```python
from build123d import *

# Parameters (mm, degrees)
SKETCH_1_R          = 10
EXTRUDE_1_DEPTH     = 5.5
SKETCH_2_R          = 6
EXTRUDE_2_DEPTH     = 5
SKETCH_3_R          = 3
EXTRUDE_3_DEPTH     = 1.5
SKETCH_4_R          = 4
EXTRUDE_4_DEPTH     = 10
CHAMFER_1_SIZE      = 1
SKETCH_5_W          = 2
SKETCH_5_H          = 20
CUT_EXTRUDE_1_DEPTH = 2.5


with BuildPart() as part:
    # 草图1 → 凸台-拉伸1 (new body)
    with BuildSketch(Plane.XY):
        Circle(SKETCH_1_R)
    extrude(amount=EXTRUDE_1_DEPTH)

    # 草图2 → 凸台-拉伸2 (add)
    with BuildSketch(Plane.XY.offset(5.5)):
        Circle(SKETCH_2_R)
    extrude(amount=EXTRUDE_2_DEPTH)

    # 草图3 → 凸台-拉伸3 (add)
    with BuildSketch(Plane.XY.offset(10.5)):
        Circle(SKETCH_3_R)
    extrude(amount=EXTRUDE_3_DEPTH)

    # 草图4 → 凸台-拉伸4 (add)
    with BuildSketch(Plane.XY.offset(12)):
        Circle(SKETCH_4_R)
    extrude(amount=EXTRUDE_4_DEPTH)

    # 倒角1
    chamfer_1_edges = [part.edges().sort_by_distance(p)[0] for p in [
        (-4, 0, 12),
        (-4, 0, 22),
    ]]
    chamfer(chamfer_1_edges, length=CHAMFER_1_SIZE - 0.0001)  # a hair under: the kernel refuses the full size

    # 草图5 → 切除-拉伸-薄壁1 (cut)
    with BuildSketch(Plane(origin=(0, 0, 0), x_dir=(-1, 0, 0), z_dir=(0, 0, -1))):
        Rectangle(SKETCH_5_W, SKETCH_5_H)
    extrude(amount=-CUT_EXTRUDE_1_DEPTH, mode=Mode.SUBTRACT)


solid = part.part
```
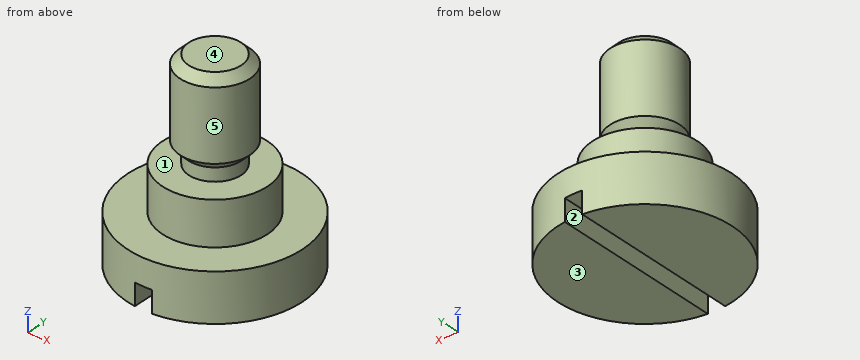
Here's how the part is built. I have some questions about the finished solid (model axes, mm). Face numbers are marked on the shaded views. A direction names the side the tool comes from. Coordinates: 2 decimals unless noted, no trailing zeros. Write each loop counter-clockwise with the first axis right and the second up, starting at its lowest first coordinate (ties: lowest second). Pieces come first, ordered by that corner, then holes. Notation, with made-up numbers: (59.5, 26) - (85.5, 26) arc R30 cw to (85.5, 57) - close; hole circle Ø3 at (-17.75, 61). An arc over 180 degrees is marked (long way). One line per item, written item: value.
1) We'd pull the mould along Z, two halves only. Please class the marked faces 1, 2 and 3: pulls with the +Z half, pulls with the -Z half, needs draft (parallel to the pull), parting line crosses it, or undercut.
Model answer:
face 1: undercut
face 2: needs draft
face 3: pulls with the -Z half
2) Suppose I cut it at D-D on z = 3. Write out the boundary of the cut face in (x, y).
Model answer:
outline: circle Ø20 at (0, 0)
3) On a 3-axis mill with a long thin cutter (end or side, diameter ignored), from which of +Z, -Z, +X, -X, +Y, -Y can I reach the whole of each face in a straight line? I mean the marked faces 4 and 5. Say none if no direction works.
Model answer:
face 4: +Z, +X, -X, +Y, -Y
face 5: +Z
4) Suppose I cut it at C-C on z = 14.5. Write out the boundary of the cut face in (x, y), and give its area (3 significant figures).
Model answer:
outline: circle Ø8 at (0, 0)
area: 50.3 mm²
5) I need wall thicknesses on line 1 along X through (y, z) = (-8, 2.25); line 2 along Z through (x, y) = (7.25, -4.5); line 3 along Z through (x, y) = (-2, -3.75). Which ranges of each line are inside material? Lowest first, please.
Model answer:
line 1: x = -6 to -1, 1 to 6
line 2: z = 0 to 5.5
line 3: z = 0 to 10.5
6) I'm going to push flat-ended pins straight in: P1, Ø1.2, axis at y = -1, z = 1, coming from the -X side; P2, Ø1, axis at y = 3, z = 14.5, coming from the -X side; P3, Ø1, axis at x = -0.5, z = 9, coming from the +Y side. Where does each tip first touch, or does it pass through?
Model answer:
P1: stops at x = -9.99
P2: stops at x = -3.12
P3: stops at y = 6
